Source: three-view drawing plus pictorial views. Frame: mm from the lowest corner of the part. A direction names the side the tool comes from. Give positions to 0.01 mm unless a question says otherwise; leave off trailing zeros. Write each loop counter-clockwise with the first axis right and the second up, starting at its lowest first coordinate (ties: lowest second). Pieces come first, ordered by that corner, then holes.
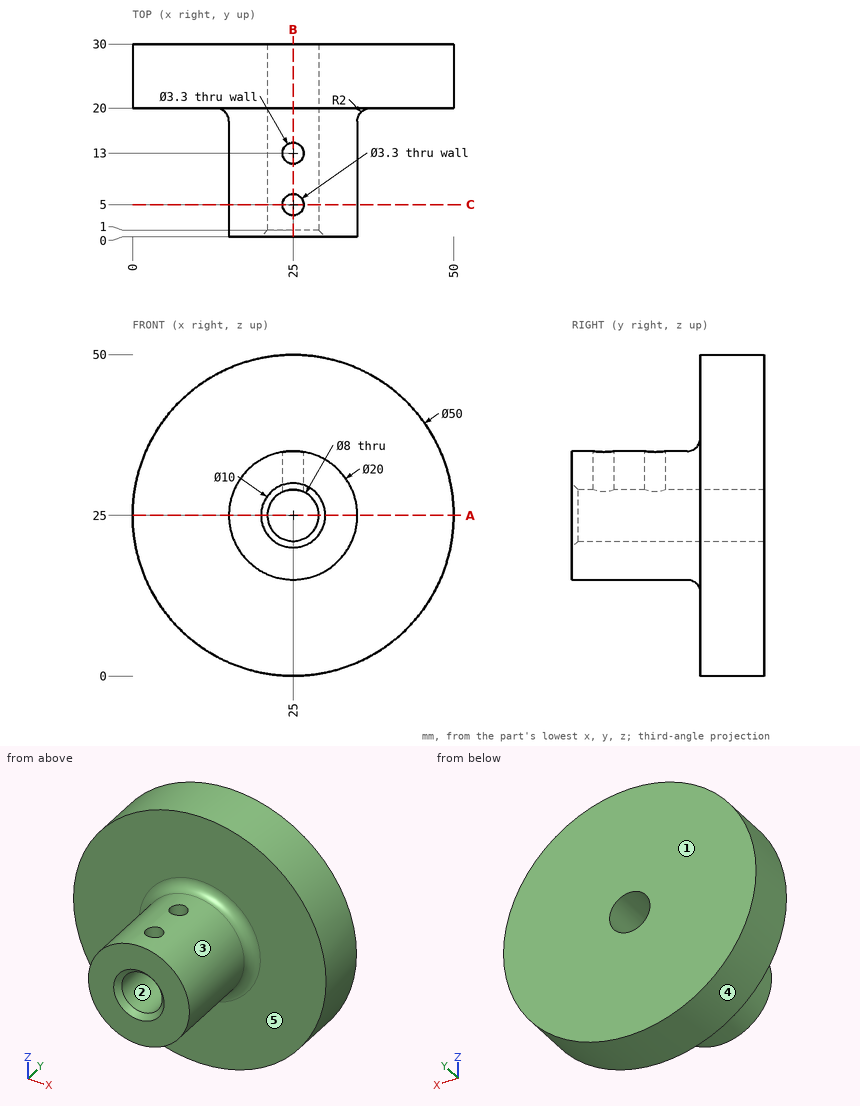
Q1. Section C-C on y = 5. Output: boundary loops of the cut face in (x, z), plus the area to 3 significant figures.
Filled sheet:
outline: (23.35, 28.64) - (23.35, 34.86) arc R10 ccw (long way) to (26.65, 34.86) - (26.65, 28.64) arc R4 cw (long way) to start
area: 244 mm2
Q2. Pin query (flat end, axial travel): P1, Ø2, axis at y = 18, z = 25.5, coming from the -X side; P2, Ø10.5, axis at x = 25, z = 25, coming from the +Y side; P3, Ø10, axis at x = 36, y = 24, coming from the +Z side; P4, Ø1, axis at x = 27.5, y = 26, coming from the -Z side. Return the tip coordinate at first contact, or that it passes through.
Filled sheet:
P1: stops at x = 14.74
P2: stops at y = 30
P3: stops at z = 49.27
P4: stops at z = 0.08
Q3. Pull-direction query (Z, two-part tool) for the marked faces 1, 2 and 3; classes: released by +Z, released by -Z, zero draft, split by the parting line, or undercut.
Filled sheet:
face 1: zero draft
face 2: undercut
face 3: split by the parting line
Q4. Ray query, line 1 along X through (y, z) = (8, 25); line 2 along Z through (x, y) = (25, 23); line 3 along Y through (x, z) = (33.5, 48). Return the intervals inside material, ascending.
Filled sheet:
line 1: x = 15 to 21, 29 to 35
line 2: z = 0 to 21, 29 to 50
line 3: y = 20 to 30
Q5. Section B-B on x = 25. Output: boundary loops of the cut face in (y, z).
Filled sheet:
outline: (0, 15) - (18, 15) arc R2 cw to (20, 13) - (20, 0) - (30, 0) - (30, 21) - (1, 21) - (0, 20) - close; (0, 30) - (1, 29) - (3.35, 29) - (3.35, 35) - (0, 35) - close; (6.65, 29) - (11.35, 29) - (11.35, 35) - (6.65, 35) - close; (14.65, 29) - (30, 29) - (30, 50) - (20, 50) - (20, 37) arc R2 cw to (18, 35) - (14.65, 35) - close
Q6. Access query for the marked faces 4 and 5. Directions: +Z, -Z, +X, -X, +Y, -Y. A direction counts if a zero-diameter tool reaches every point of the face in a straight line with its end or side. Return the directions, or none.
Filled sheet:
face 4: +Y, -Y
face 5: -Y
Q7. Section A-A on z = 25. Output: boundary loops of the cut face in (x, y).
Filled sheet:
outline: (0, 20) - (13, 20) arc R2 cw to (15, 18) - (15, 0) - (20, 0) - (21, 1) - (21, 30) - (0, 30) - close; (29, 1) - (30, 0) - (35, 0) - (35, 18) arc R2 cw to (37, 20) - (50, 20) - (50, 30) - (29, 30) - close
